```python
from build123d import *

# Parameters (mm, degrees)
CROQUIS1_W              = 12
CROQUIS1_H              = 12.1
SALIENTE_EXTRUIR1_DEPTH = 11.6
CROQUIS2_W              = 12
CROQUIS2_H              = 3
SALIENTE_EXTRUIR2_DEPTH = 2.2
CROQUIS3_R              = 0.6
SALIENTE_EXTRUIR3_DEPTH = 3.6


with BuildPart() as part:
    # Croquis1 → Saliente-Extruir1 (new body)
    with BuildSketch(Plane(origin=(0, 0, 0), x_dir=(1, 0, 0), z_dir=(0, 1, 0))):
        Rectangle(CROQUIS1_W, CROQUIS1_H)
    extrude(amount=SALIENTE_EXTRUIR1_DEPTH)

    # Croquis2 → Saliente-Extruir2 (add)
    with BuildSketch(Plane(origin=(0, 11.6, 0), x_dir=(1, 0, 0), z_dir=(0, 1, 0))):
        Rectangle(CROQUIS2_W, CROQUIS2_H)
    extrude(amount=SALIENTE_EXTRUIR2_DEPTH)

    # Croquis3 → Saliente-Extruir3 (add)
    with BuildSketch(Plane.XZ):
        with Locations(Location((-2.75, -1.35, 0), (0, 0, 270))):
            Circle(CROQUIS3_R)
        with Locations(Location((0.75, 3.75, 0), (0, 0, 270))):
            Circle(CROQUIS3_R)
        with Locations(Location((4.25, -1.35, 0), (0, 0, 270))):
            Circle(CROQUIS3_R)
    extrude(amount=SALIENTE_EXTRUIR3_DEPTH)


solid = part.part
```
Build history of the part. All positions in model axes, mm. A direction names the side the tool comes from. Round coordinates to 2 decimals unless told otherwise and drop trailing zeros. Loops run counter-clockwise (first coordinate to the right, second up) from the corner with the lowest first, then second, coordinate; pieces in that order, holes last.
Item 1: Two-plate mould, pull along X, no slides. Class faces 1 (the face through (-2.244, -1.775, -1.673)), 2 (the face through (0, 6, 6.05)), 3 (the face through (-6, 7, 0)): released by +X, released by -X, zero draft, split by the parting line, or undercut.
Item 2: Saw through at A-A (x = 2.25). List the corners of the cut face in (y, z), then the cut area to 3 significant figures.
Item 3: Saw through at D-D (x = -2.75). List the corners of the cut face in (y, z).
Item 4: Drill centre lines: line 1 along Y through (x, z) = (3.5, 1.25); line 2 along Y through (x, z) = (-3, -3.75); line 3 along X through (y, z) = (-2.5, 3.25). Where is each one in solid material? Low to high.
Item 5: Which spindle directions (+Z, -Z, +X, -X, +Y, -Y) get a long thin tool onto all of the face, cutting with end or side? Do faces 4 (the face through (6, 7, 0)), 5 (the face through (0, 6, -6.05)), 6 (the face through (3.72, -1.77, -1.63)), 7 (the face through (0, 13, 1.5)), 8 (the face through (0, 13, -1.5)). Say none if no direction does.
Item 6: Saw through at C-C (y = -1). List the corners of the cut face in (x, z), then the cut area to 3 significant figures.
Item 7: Saw through at B-B (z = 3.75). List the corners of the cut face in (x, y).
Item 8: Pin check, flat tips, straight feed: P1, Ø3.5, axis at x = 0.5, z = 3.5, coming from the +Y side; P2, Ø2.5, axis at x = 3, y = 13, coming from the +Z side. Stop position of each tip, or through.
Worked answers:
1. face 1: undercut
1. face 2: zero draft
1. face 3: released by -X
2. outline: (0, -6.05) - (11.6, -6.05) - (11.6, -1.5) - (13.8, -1.5) - (13.8, 1.5) - (11.6, 1.5) - (11.6, 6.05) - (0, 6.05) - close
2. area: 147 mm2
3. outline: (-3.6, -1.95) - (0, -1.95) - (0, -6.05) - (11.6, -6.05) - (11.6, -1.5) - (13.8, -1.5) - (13.8, 1.5) - (11.6, 1.5) - (11.6, 6.05) - (0, 6.05) - (0, -0.75) - (-3.6, -0.75) - close
4. line 1: y = 0 to 13.8
4. line 2: y = 0 to 11.6
4. line 3: x = 0.42 to 1.08
5. face 4: +Z, -Z, +X, +Y, -Y
5. face 5: -Z, +X, -X, +Y, -Y
5. face 6: -Y
5. face 7: +Z, +X, -X, +Y
5. face 8: -Z, +X, -X, +Y
6. outline: circle Ø1.2 at (-2.75, -1.35); circle Ø1.2 at (0.75, 3.75); circle Ø1.2 at (4.25, -1.35)
6. area: 3.39 mm2
7. outline: (-6, 0) - (0.15, 0) - (0.15, -3.6) - (1.35, -3.6) - (1.35, 0) - (6, 0) - (6, 11.6) - (-6, 11.6) - close
8. P1: stops at y = 11.6
8. P2: stops at z = 1.5
